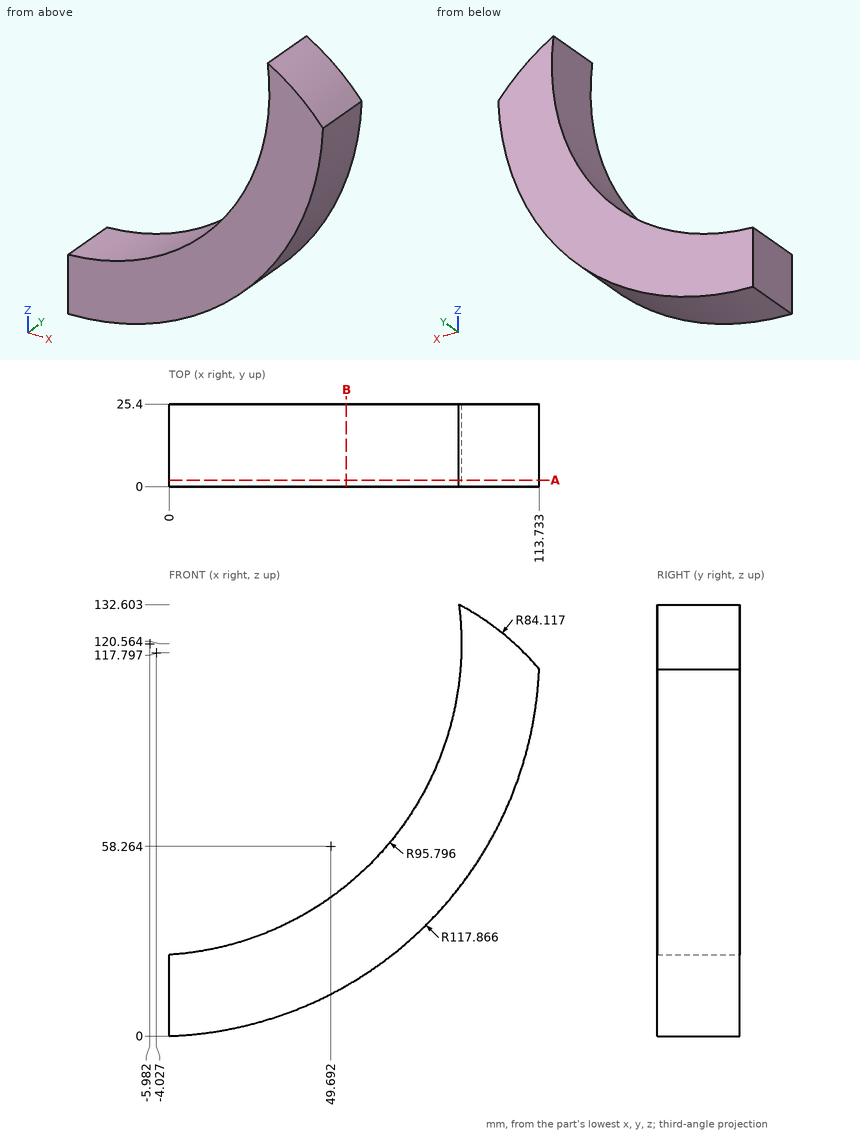
Could you check a few things on this drawing? It's one solid part, dimensions in mm from its lowest x, y, z. Give positions to 0.01 mm unless a question says otherwise; leave off trailing zeros. Loops run counter-clockwise (first coordinate to the right, second up) from the corner with the lowest first, then second, coordinate; pieces in that order, holes last. Notation, with made-up numbers: M 76.25,55 L 112.25,55 A14 cw 112.25,61 Z; hole C 9,47 d3. An arc over 180 degrees is marked long. One line per question, with ' | ' between items. Start each with the question number.
Q1. If we section it at B-B (x = 54.5): Please give me the cut outline in (y, z) (1 decimal), plus the area to 3 significant figures.
Q2. For pin 1 Ø1 at (y, z) = (6.5, 99.5) entering from +X; pin 2 Ø3 at (x, y) = (28, 18) entering from +Z; pin 3 Ø2 at (y, z) = (7.5, 37) entering from +X, each with a flat end and sliding along its axis, tell me the tip position at first contact or that it passes through.
Q3. If I drill on line 1 (X direction, y = 4.25, z = 104); line 2 (Z direction, x = 26, y = 3.25) (1 decimal); line 3 (Z direction, x = 32, y = 20.75), over which ranges is the centre line in solid material (lowest first)? Write a range as from..to.
Q4. If we section it at A-A (y = 2): Please give me the cut outline in (x, z) (1 decimal).
Computed:
1) outline: M 0,15.5 L 25.4,15.5 L 25.4,46.3 L 0,46.3 Z | area: 782 mm²
2) pin 1: stops at x = 112.49 | pin 2: stops at z = 31.58 | pin 3: stops at x = 82.72
3) line 1: x = 88.37..113.03 | line 2: z = 3.8..30.3 | line 3: z = 5.57..32.62
4) outline: M 0,0 A117.9 ccw 113.7,112.8 A84.1 ccw 89.1,132.6 A95.8 cw 0,25 Z
